```python
from build123d import *

# Parameters (mm, degrees)
SKETCH2_R           = 56.85
SKETCH2_R_2         = 44.5
BOSS_EXTRUDE1_DEPTH = 1.2
SKETCH3_R           = 56.85
BOSS_EXTRUDE2_DEPTH = 10
SKETCH4_R           = 2.65
CUT_EXTRUDE1_DEPTH  = 12.2
SKETCH5_R           = 7.5
CUT_EXTRUDE2_DEPTH  = 12.2
CUT_EXTRUDE4_DEPTH  = 11
SKETCH7_W           = 20
SKETCH7_H           = 5
BOSS_EXTRUDE3_DEPTH = 1
BOSS_EXTRUDE4_DEPTH = 1
CIRPATTERN1_COUNT   = 6
SKETCH9_R           = 4.35
CUT_EXTRUDE5_DEPTH  = 5.4
CHAMFER1_SIZE       = 1
CHAMFER2_SIZE       = 1


with BuildPart() as part:
    # Sketch2 → Boss-Extrude1 (new body)
    with BuildSketch(Plane(origin=(0, 0, 0), x_dir=(1, 0, 0), z_dir=(0, 1, 0))):
        Circle(SKETCH2_R)
        Circle(SKETCH2_R_2, mode=Mode.SUBTRACT)
    extrude(amount=BOSS_EXTRUDE1_DEPTH)

    # Sketch3 → Boss-Extrude2 (add)
    with BuildSketch(Plane(origin=(0, 1.2, 0), x_dir=(1, 0, 0), z_dir=(0, 1, 0))):
        Circle(SKETCH3_R)
    extrude(amount=BOSS_EXTRUDE2_DEPTH)

    # Sketch4 → Cut-Extrude1 (cut, through all)
    with BuildSketch(Plane(origin=(0, 11.2, 0), x_dir=(1, 0, 0), z_dir=(0, 1, 0))):
        with Locations((-13.005657016, 48.537772771)):
            Circle(SKETCH4_R)
        with Locations((48.537772771, 13.005657016)):
            Circle(SKETCH4_R)
        with Locations((13.005657016, -48.537772771)):
            Circle(SKETCH4_R)
        with Locations((-48.537772771, -13.005657016)):
            Circle(SKETCH4_R)
    extrude(amount=-CUT_EXTRUDE1_DEPTH, mode=Mode.SUBTRACT)

    # Sketch5 → Cut-Extrude2 (cut, through all)
    with BuildSketch(Plane(origin=(0, 11.2, 0), x_dir=(1, 0, 0), z_dir=(0, 1, 0))):
        Circle(SKETCH5_R)
    extrude(amount=-CUT_EXTRUDE2_DEPTH, mode=Mode.SUBTRACT)

    # Sketch6 → Cut-Extrude4 (cut, through all)
    with BuildSketch(Plane.XZ.offset(-1.2)):
        Polygon((12.845675931, 27.249363369), (10.876265015, 23.838243602), (5.505548638, 33.14059724), (-5.505548638, 33.14059724), (-10.876265015, 23.838243603), (-12.845675931, 27.249363369), (-17.175802949, 24.749363369), (-15.206392034, 21.338243603), (-25.947824787, 21.338243603), (-31.453373426, 11.802353637), (-26.082657049, 2.5), (-30.02147888, 2.5), (-30.02147888, -2.5), (-26.082657049, -2.5), (-31.453373426, -11.802353638), (-25.947824787, -21.338243603), (-15.206392034, -21.338243603), (-17.175802949, -24.749363369), (-12.845675931, -27.249363369), (-10.876265015, -23.838243603), (-5.505548638, -33.14059724), (5.505548638, -33.14059724), (10.876265015, -23.838243603), (12.845675931, -27.249363369), (17.175802949, -24.749363369), (15.206392034, -21.338243603), (25.947824787, -21.338243603), (31.453373426, -11.802353638), (26.082657049, -2.5), (30.02147888, -2.5), (30.02147888, 2.5), (26.082657049, 2.5), (31.453373426, 11.802353637), (25.947824787, 21.338243602), (15.206392034, 21.338243602), (17.175802949, 24.749363369), align=None)
        Polygon((-2.845675931, 9.928855294), (-5.235884115, 14.06881731), (5.235884115, 14.06881731), (2.845675931, 9.928855294), (7.175802949, 7.428855294), (9.566011134, 11.56881731), (14.801895249, 2.5), (10.02147888, 2.5), (10.02147888, -2.5), (14.801895249, -2.5), (9.566011134, -11.56881731), (7.175802949, -7.428855294), (2.845675931, -9.928855294), (5.235884115, -14.06881731), (-5.235884115, -14.06881731), (-2.845675931, -9.928855294), (-7.175802949, -7.428855294), (-9.566011134, -11.56881731), (-14.801895249, -2.5), (-10.02147888, -2.5), (-10.02147888, 2.5), (-14.801895249, 2.5), (-9.566011134, 11.56881731), (-7.175802949, 7.428855294), align=None, mode=Mode.SUBTRACT)
    extrude(amount=-CUT_EXTRUDE4_DEPTH, mode=Mode.SUBTRACT)

    # Sketch7 → Boss-Extrude3 (add)
    with BuildSketch(Plane(origin=(0, 11.2, 0), x_dir=(1, 0, 0), z_dir=(0, 1, 0))):
        Polygon((-17.175802949, 24.749363369), (-7.175802949, 7.428855294), (-2.845675931, 9.928855294), (-12.845675931, 27.249363369), align=None)
        Polygon((17.175802949, 24.749363369), (12.845675931, 27.249363369), (2.845675931, 9.928855294), (7.175802949, 7.428855294), align=None)
        with Locations((20.02147888, 0)):
            Rectangle(SKETCH7_W, SKETCH7_H)
        Polygon((12.845675931, -27.249363369), (17.175802949, -24.749363369), (7.175802949, -7.428855294), (2.845675931, -9.928855294), align=None)
        Polygon((-17.175802949, -24.749363369), (-12.845675931, -27.249363369), (-2.845675931, -9.928855294), (-7.175802949, -7.428855294), align=None)
        with Locations((-20.02147888, 0)):
            Rectangle(SKETCH7_W, SKETCH7_H)
    extrude(amount=-BOSS_EXTRUDE3_DEPTH)

    # Sketch8 → Boss-Extrude4 (add)
    with BuildSketch(Plane(origin=(0, 11.2, 0), x_dir=(1, 0, 0), z_dir=(0, 1, 0))):
        Polygon((5.542562584, -14.00470728), (-5.542562584, -14.00470728), (-11.085125168, -23.60470728), (-5.542562584, -33.20470728), (5.542562584, -33.20470728), (11.085125168, -23.60470728), align=None)
        Polygon((5.196152423, -14.60470728), (-5.196152423, -14.60470728), (-10.392304845, -23.60470728), (-5.196152423, -32.60470728), (5.196152423, -32.60470728), (10.392304845, -23.60470728), align=None, mode=Mode.SUBTRACT)
    boss_extrude4 = extrude(amount=-BOSS_EXTRUDE4_DEPTH)

    # CirPattern1: Boss-Extrude4 ×6 about axis
    cirpattern1_axis = Axis((0, 0, 0), (0, 1, 0))
    for i in range(1, CIRPATTERN1_COUNT):
        add(boss_extrude4.rotate(cirpattern1_axis, i * 360 / CIRPATTERN1_COUNT))

    # Sketch9 → Cut-Extrude5 (cut)
    with BuildSketch(Plane(origin=(0, 11.2, 0), x_dir=(1, 0, 0), z_dir=(0, 1, 0))):
        with Locations((-13.005657016, 48.537772771)):
            Circle(SKETCH9_R)
        with Locations((48.537772771, 13.005657016)):
            Circle(SKETCH9_R)
        with Locations((13.005657016, -48.537772771)):
            Circle(SKETCH9_R)
        with Locations((-48.537772771, -13.005657016)):
            Circle(SKETCH9_R)
    extrude(amount=-CUT_EXTRUDE5_DEPTH, mode=Mode.SUBTRACT)

    # Chamfer1
    chamfer1_edges = [part.edges().sort_by_distance(p)[0] for p in [
        (-44.5, 0, 0),
        (-56.85, 0, 0),
    ]]
    chamfer(chamfer1_edges, length=CHAMFER1_SIZE)

    # Chamfer2
    chamfer2_edges = [part.edges().sort_by_distance(p)[0] for p in [
        (-7.5, 11.2, 0),
    ]]
    chamfer(chamfer2_edges, length=CHAMFER2_SIZE)


solid = part.part
```
Check sheet for the modelled part. Datum: model origin and axes. Units: mm. A direction names the side the tool comes from. Coordinates: 2 decimals unless noted, no trailing zeros. Order: outer loops, then holes, each group sorted by start corner. A loop starts at its lowest first (then second) coordinate and runs counter-clockwise, first axis right, second up. Notation, with made-up numbers: (-12, -30) -> (28, -30) arc R22 ccw to (28, -5) -> close; hole circle Ø7 at (2, -12.75). An arc over 180 degrees is marked (long way). Write item = value, one per line. Start each with the question number.
1) Access from +Z, -Z, +X, -X, +Y, -Y to the whole of each face (thin tool, end or side, straight path). Record for faces 1 (the flat face through (-12.684, 10.707, -7.239)), 2 (the flat face through (-8.153, 5.637, 28.555)), 3 (the flat face through (16, 5.8, 48)).
2) Material ranges on L1, parallel to Z at x = 0, y = 3.5; L2, parallel to Z at x = 11, y = 5.5; L3, parallel to Z at x = 14, y = 10, recorded low to high.
3) Go/stop test with flat-tipped pins: P1, Ø1, axis at y = 1, z = -26.5, coming from the -X side; P2, Ø6, axis at y = 2, z = 29, coming from the +X side; P3, Ø3, axis at x = 27.5, y = 5, coming from the -Z side. Record where each tip stops, or that it passes through.
4) Cross-section at A-A (z = 0). Enter the section's corners in (x, y), then the cut area to 3 significant figures.
5) Cross-section at B-B (x = 0). State how many separate pieces and enclosed holes the cut face has, then the cut area to 3 significant figures.
Ans:
q1.face_1 = +Y, -Y
q1.face_2 = -Y
q1.face_3 = +Y
q2.L1 = -56.85 to -33.14, -14.07 to -7.5, 7.5 to 14.07, 33.14 to 56.85
q2.L2 = -55.78 to -24.05, -9.09 to -2.5, 2.5 to 9.09, 24.05 to 46.81, 50.27 to 55.78
q2.L3 = -55.1 to -26.58, -3.89 to -2.5, 2.5 to 3.89, 26.58 to 44.3, 52.77 to 55.1
q3.P1 = -50.56
q3.P2 = 50.56
q3.P3 = -50.56
q4.outline = (-56.85, 1) -> (-55.85, 0) -> (-45.5, 0) -> (-44.5, 1) -> (-44.5, 1.2) -> (-30.02, 1.2) -> (-30.02, 10.2) -> (-10.02, 10.2) -> (-10.02, 1.2) -> (-7.5, 1.2) -> (-7.5, 10.2) -> (-8.5, 11.2) -> (-56.85, 11.2) -> close; (7.5, 1.2) -> (10.02, 1.2) -> (10.02, 10.2) -> (30.02, 10.2) -> (30.02, 1.2) -> (44.5, 1.2) -> (44.5, 1) -> (45.5, 0) -> (55.85, 0) -> (56.85, 1) -> (56.85, 11.2) -> (8.5, 11.2) -> (7.5, 10.2) -> close
q4.area = 654 mm²
q5.separate_pieces = 4
q5.enclosed_holes = 0
q5.area = 634 mm²
